Input: dimensioned drawing with shaded views. Units: mm. Origin: part minimum x, y, z. A direction names the side the tool comes from. Round coordinates to 2 decimals unless told otherwise and drop trailing zeros. Loops run counter-clockwise (first coordinate to the right, second up) from the corner with the lowest first, then second, coordinate; pieces in that order, holes last.
Item 1: Access query for the marked faces 1 and 2. Directions: +Z, -Z, +X, -X, +Y, -Y. A direction counts if a zero-diameter tool reaches every point of the face in a straight line with its end or side. Return the directions, or none.
Item 2: First-contact query: P1, Ø3, axis at x = 2, z = 2.5, coming from the +Y side; P2, Ø1, axis at x = 4.5, z = 3, coming from the +Y side. Flat tips, straight axial feed; report the tip coordinate or a pass-through.
Item 3: Section query B-B on z = 4.5. Return loops of the section in (x, y), then the cut area to 3 significant figures.
Item 4: Ray query, L1, parallel to Z at x = 12.25, y = 9; L2, parallel to Y at x = 2.5, z = 1.5; L3, parallel to Y at x = 8.5, z = 0.5. Return the intervals inside material, ascending.
Item 5: Section query A-A on z = 2. Return loops of the section in (x, y), then the cut area to 3 significant figures.
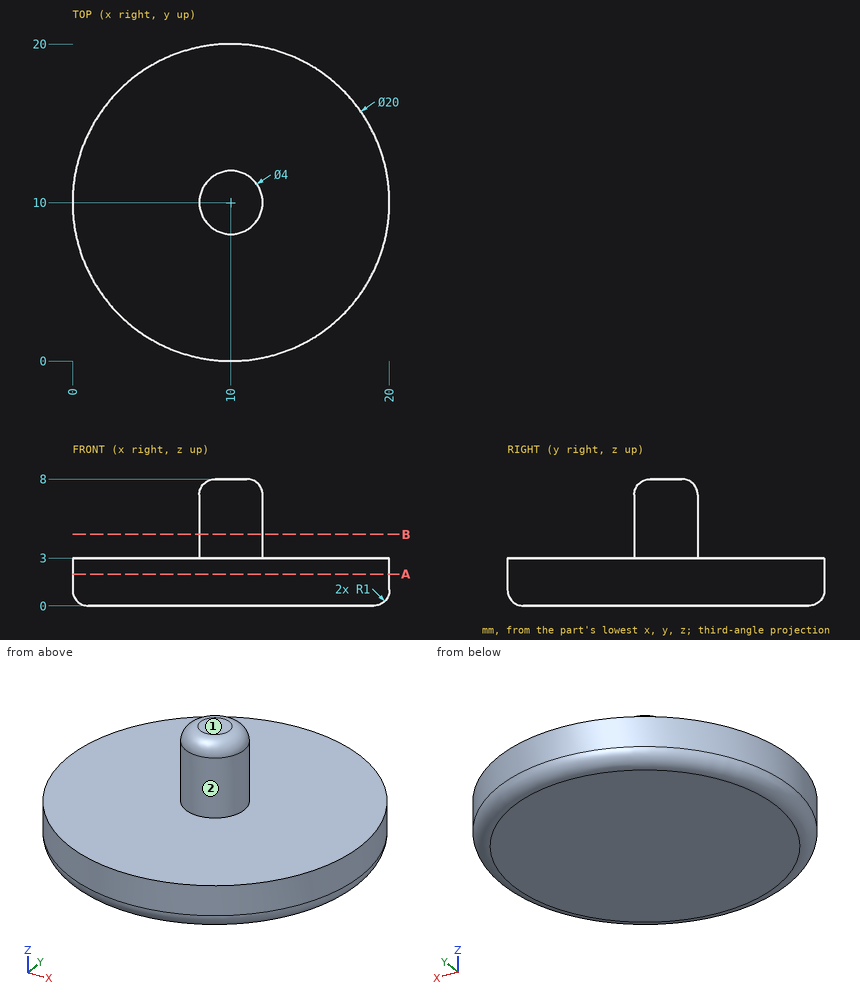
Data:
1. face 1: +Z, +X, -X, +Y, -Y
1. face 2: +Z
2. P1: stops at y = 17.6
2. P2: stops at y = 18.66
3. outline: circle Ø4 at (10, 10)
3. area: 12.6 mm2
4. L1: z = 0 to 3
4. L2: y = 3.39 to 16.61
4. L3: y = 0.25 to 19.75
5. outline: circle Ø20 at (10, 10)
5. area: 314 mm2
